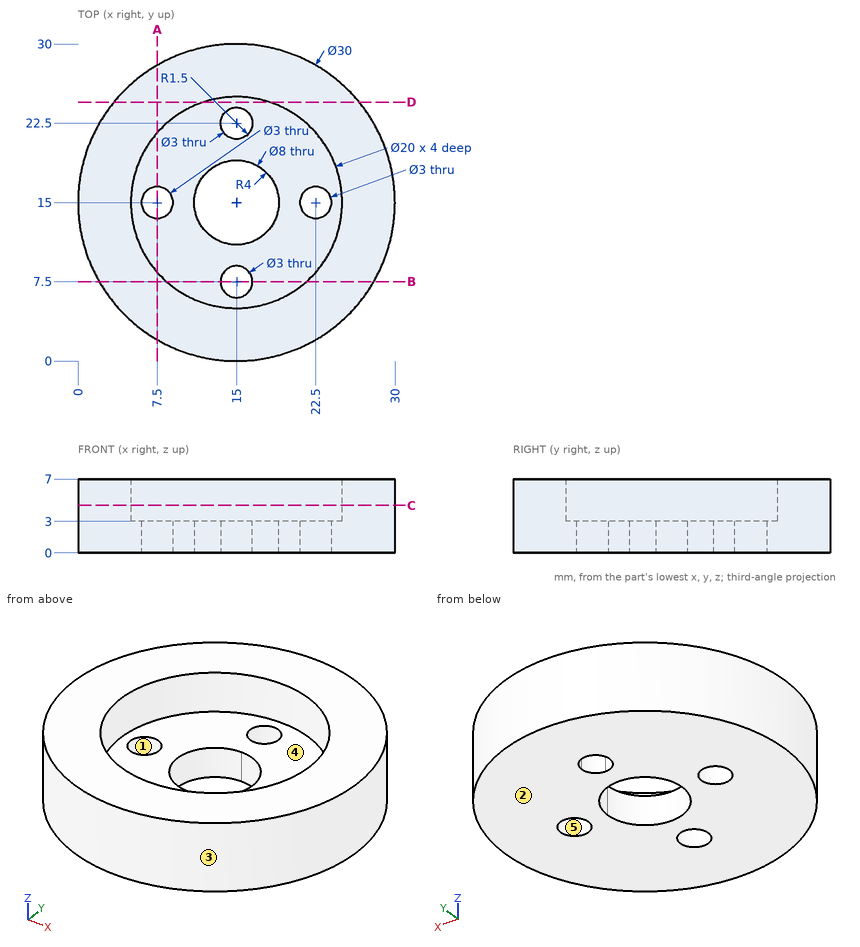
Design review of the part shown in the three views and the two pictorial views. Dimensions are in mm from the part's minimum x, y and z. A direction names the side the tool comes from. Coordinates: 2 decimals unless noted, no trailing zeros. Loops run counter-clockwise (first coordinate to the right, second up) from the corner with the lowest first, then second, coordinate; pieces in that order, holes last. Notation, with made-up numbers: (67, 80) - (78, 80) arc R22 cw to (78, 105) - close; hole circle Ø9 at (63, -26). An arc over 180 degrees is marked (long way). Use a Markdown table: item, result. Add a question column.
Item 1: Tool access review of the marked faces 4 and 5: name each direction out of +Z, -Z, +X, -X, +Y, -Y from which nothing blocks a thin tool from reaching the whole face with its end or side.
Item 2: We need section A-A (x = 7.5). Give the boundary of the cut face in (y, z).
Item 3: We need section D-D (y = 24.5). Give the boundary of the cut face in (x, z), and give its area (3 significant figures).
Item 4: For line 1 (Y direction, x = 15, z = 1.5); line 2 (Z direction, x = 20.75, y = 11); line 3 (X direction, y = 8.5, z = 4.75), list the stretches that pass through material, from the lowest coordinate up.
Item 5: Mouldability with a two-part tool opening along Y and no side actions: class the marked faces 1, 2 and 3 as pulls with the +Y half, pulls with the -Y half, needs draft (parallel to the pull), parting line crosses it, or undercut.
Item 6: Insertion check: pin 1 Ø2.5 at (x, y) = (15, 7.5) entering from -Z; pin 2 Ø1 at (y, z) = (21.5, 1) entering from +X; pin 3 Ø1 at (x, z) = (13.5, 2.5) entering from -Y; pin 4 Ø6 at (x, y) = (11, 14.5) entering from +Z. Each pin has a flat end and moves straight along its axis. Give the tip position at first contact, or say it passes through.
Item 7: We need section C-C (z = 4.5). Give the boundary of the cut face in (x, y), and give its area (3 significant figures).
Results list:
| question | item | result |
|---|---|---|
| 1 | face 4 | +Z |
| 1 | face 5 | +Z, -Z |
| 2 | outline | (2.01, 0) - (13.5, 0) - (13.5, 3) - (8.39, 3) - (8.39, 7) - (2.01, 7) - close; (16.5, 0) - (27.99, 0) - (27.99, 7) - (21.61, 7) - (21.61, 3) - (16.5, 3) - close |
| 3 | outline | (3.39, 0) - (26.61, 0) - (26.61, 7) - (18.12, 7) - (18.12, 3) - (11.88, 3) - (11.88, 7) - (3.39, 7) - close |
| 3 | area | 138 mm^2 |
| 4 | line 1 | y = 0 to 6, 9 to 11, 19 to 21, 24 to 30 |
| 4 | line 2 | z = 0 to 3 |
| 4 | line 3 | x = 1.48 to 7.4, 22.6 to 28.52 |
| 5 | face 1 | undercut |
| 5 | face 2 | needs draft |
| 5 | face 3 | parting line crosses it |
| 6 | pin 1 | passes through |
| 6 | pin 2 | stops at x = 28.75 |
| 6 | pin 3 | stops at y = 0.03 |
| 6 | pin 4 | stops at z = 3 |
| 7 | outline | circle Ø30 at (15, 15); hole circle Ø20 at (15, 15) |
| 7 | area | 393 mm^2 |
